Design review of the part built by this model. Coordinates are the model's own, in mm. Round coordinates to 2 decimals unless told otherwise and drop trailing zeros. Write each loop counter-clockwise with the first axis right and the second up, starting at its lowest first coordinate (ties: lowest second). Pieces come first, ordered by that corner, then holes. Notation, with made-up numbers: (79.25, 79.5) -> (107.25, 79.5) arc R17 ccw to (107.25, 108.5) -> close; hole circle Ø10 at (40.25, 75.25). An arc over 180 degrees is marked (long way). Write item = value, one per line. Start each with the question number.
Item 1: Add section B-B, the plane z = -15. State the section outline as (x, y) points.
Item 2: To check wall thickness, follow L1, parallel to Z at x = 2.4, y = -2.5; L2, parallel to Z at x = 2.45, y = -21.5; L3, parallel to Y at x = 3.15, z = 23. State the ranges of each line that lie inside material, in increasing order.
Item 3: Add section A-A, the plane x = 1.85. State the section outline as (y, z) points.
Item 4: Add section C-C, the plane y = -36.5. State the section outline as (x, z) points.
Item 5: For pin 1 Ø2 at (x, y) = (1, -4) entering from -Z; pin 2 Ø1.2 at (x, z) = (1, 31) entering from +Y; pin 3 Ø2 at (x, z) = (2.5, 24.5) entering from -Y, all flat-tipped, find the tip position at first contact; note any pin that passes through.
Item 6: Add section D-D, the plane z = -4. State the section outline as (x, y) points, then the cut area to 3 significant figures.
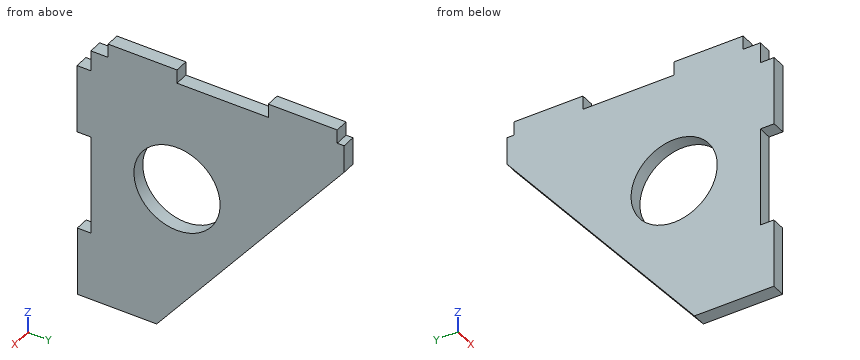
from build123d import *

# Parameters (mm, degrees)
SKETCH1_R           = 12.5
BOSS_EXTRUDE1_DEPTH = 4


with BuildPart() as part:
    # Sketch1 → Boss-Extrude1 (new body)
    with BuildSketch(Plane(origin=(0, 0, 0), x_dir=(0, 0, -1), z_dir=(1, 0, 0))):
        Polygon((-32.145071831, 34.052951323), (-32.145071831, 14.052951323), (-28.145071831, 14.052951323), (-28.145071831, -12.409790693), (-32.145071831, -12.409790693), (-32.145071831, -32.409790693), (-28.145071831, -32.409790693), (-28.145071831, -37.409790693), (-22.145071831, -37.409790693), (-22.145071831, -41.409790693), (-2.145071831, -41.409790693), (-2.145071831, -37.409790693), (26.854928169, -37.409790693), (26.854928169, -41.322671818), (46.854928169, -41.322671818), (46.854928169, -18.308632295), (-20.145071831, 36.057032999), (-28.145071831, 36.057032999), (-28.145071831, 34.052951323), align=None)
        with Locations((3.793770472, -12.409790693)):
            Circle(SKETCH1_R, mode=Mode.SUBTRACT)
    extrude(amount=BOSS_EXTRUDE1_DEPTH)


solid = part.part
Result set:
q1.outline = (0, -37.41) -> (4, -37.41) -> (4, -17.95) -> (0, -17.95) -> close; (0, -6.87) -> (4, -6.87) -> (4, 7.54) -> (0, 7.54) -> close
q2.L1 = -27.37 to -11.41, 3.83 to 28.15
q2.L2 = -46.85 to -12.37, 4.79 to 32.15
q2.L3 = -37.41 to 36.06
q3.outline = (-41.41, 2.15) -> (-37.41, 2.15) -> (-37.41, -26.85) -> (-41.32, -26.85) -> (-41.32, -46.85) -> (-18.31, -46.85) -> (36.06, 20.15) -> (36.06, 28.15) -> (34.05, 28.15) -> (34.05, 32.15) -> (14.05, 32.15) -> (14.05, 28.15) -> (-12.41, 28.15) -> (-12.41, 32.15) -> (-32.41, 32.15) -> (-32.41, 28.15) -> (-37.41, 28.15) -> (-37.41, 22.15) -> (-41.41, 22.15) -> close; hole circle Ø25 at (-12.41, -3.79)
q4.outline = (0, -46.85) -> (4, -46.85) -> (4, 28.15) -> (0, 28.15) -> close
q5.pin_1 = -30.45
q5.pin_2 = 34.05
q5.pin_3 = -37.41
q6.outline = (0, -37.41) -> (4, -37.41) -> (4, -24.91) -> (0, -24.91) -> close; (0, 0.09) -> (4, 0.09) -> (4, 16.47) -> (0, 16.47) -> close
q6.area = 116 mm²
